The model under review builds one solid part; all positions refer to its coordinate system, in mm. A direction names the side the tool comes from. Round coordinates to 2 decimals unless told otherwise and drop trailing zeros. Order: outer loops, then holes, each group sorted by start corner. A loop starts at its lowest first (then second) coordinate and runs counter-clockwise, first axis right, second up. Notation, with made-up numbers: M 35.5,65 L 68.5,65 A10 ccw 68.5,81 Z; hole C 46.25,52 d9. An arc over 180 degrees is marked long. Answer as a JSON object with one key per item and string values. Group by question number.
1. Clearance check with flat-ended pins moving along their axes: P1, Ø2.5, axis at x = 14, z = 5.5, coming from the +Y side; P2, Ø10, axis at x = -13.5, z = 5.5, coming from the +Y side; P3, Ø8.5, axis at x = 12, z = -3, coming from the +Y side. State where each tip first meets the part, or that it passes through.
2. To check wall thickness, follow probe 1 along X at (y, z) = (1.75, 6.75); probe 2 along Z at (x, y) = (21, 1.5); probe 3 along Y at (x, z) = (-6.5, 7.5). State the ranges of each line that lie inside material, in increasing order. Write a range as [from, to].
3. Add section C-C on y = 3. Give the number of separate pieces and of enclosed holes in the cut face, and give its area (3 significant figures).
4. Add section B-B on z = -5. State the section outline as (x, y) points, and give its area (3 significant figures).
5. Add section A-A on x = -6. State the section outline as (y, z) points, and give its area (3 significant figures).
6. Machinability: for faces 1 (the face through (11, 0.5, -4)), 2 (the face through (22.21, 0.99, 8.23)), 3 (the face through (-0.218, 3.288, -1.663)), which of the approach directions +Z, -Z, +X, -X, +Y, -Y give a long, thin tool a straight path to every point of the face, cutting with its end or side? Answer none if there is none.
7. Mouldability with a two-part tool opening along Z and no side actions: class faces 4 (the face through (-22.21, 0.99, -8.23)), 5 (the face through (0, 0, 0)), 6 (the face through (-22.4, 3, 8.3)), 7 (the face through (-1.375, 3.288, 1.35)) as released by +Z, released by -Z, zero draft, split by the parting line, or undercut.
```python
from build123d import *

# Parameters (mm, degrees)
BOSS_EXTRUDE1_DEPTH = 4
BOSS_EXTRUDE1_DRAFT = -1
SHELL1_T            = -0.5
SKETCH2_R           = 2
BOSS_EXTRUDE2_DEPTH = 5.5
BOSS_EXTRUDE2_TAPER = 1.5
CIRPATTERN1_COUNT   = 4
SKETCH4_R           = 1.605977431
CUT_EXTRUDE1_DEPTH  = 5.5
CUT_EXTRUDE1_DRAFT  = 1.5
RIB3_START          = -22.069744096
RIB3_DEPTH          = 20.231981802
RIB3_START_2        = 1.837762294
RIB3_2_DEPTH        = 20.231981802
RIB3_START_3        = -8.069744096
RIB3_3_DEPTH        = 6.231981802
RIB3_4_DEPTH        = 6.231981802


with BuildPart() as part:
    # Sketch1 → Boss-Extrude1 (with draft: the straight prism first)
    with BuildSketch(Plane(origin=(0, 0, 0), x_dir=(1, 0, 0), z_dir=(0, 1, 0))):
        with BuildLine():
            Line((-21.5, -8.5), (21.5, -8.5))
            ThreePointArc((21.5, -8.5), (22.207106781, -8.207106781), (22.5, -7.5))
            Line((22.5, -7.5), (22.5, 7.5))
            ThreePointArc((22.5, 7.5), (22.207106781, 8.207106781), (21.5, 8.5))
            Line((21.5, 8.5), (-21.5, 8.5))
            ThreePointArc((-21.5, 8.5), (-22.207106781, 8.207106781), (-22.5, 7.5))
            Line((-22.5, 7.5), (-22.5, -7.5))
            ThreePointArc((-22.5, -7.5), (-22.207106781, -8.207106781), (-21.5, -8.5))
        make_face()
    extrude(amount=BOSS_EXTRUDE1_DEPTH)
    # Boss-Extrude1: the draft: its side faces are tilted about the plane it starts from
    boss_extrude1_sides = [part.faces().sort_by_distance(p)[0] for p in [
        (0, 2, 8.5),
        (22.207106781, 2, 8.207106781),
        (22.5, 2, 0),
        (22.207106781, 2, -8.207106781),
        (0, 2, -8.5),
        (-22.207106781, 2, -8.207106781),
        (-22.5, 2, 0),
        (-22.207106781, 2, 8.207106781),
    ]]
    draft(boss_extrude1_sides, Plane(origin=(0, 0, 0), x_dir=(1, 0, 0), z_dir=(0, 1, 0)), BOSS_EXTRUDE1_DRAFT)

    # Shell1
    shell1_openings = [part.faces().sort_by_distance(p)[0] for p in [
        (0, 4, 0),
    ]]
    offset(amount=SHELL1_T, openings=shell1_openings, kind=Kind.INTERSECTION)

    # Sketch2 → Boss-Extrude2 (add)
    with BuildSketch(Plane(origin=(0, 0.5, 0), x_dir=(1, 0, 0), z_dir=(0, 1, 0))):
        Circle(SKETCH2_R)
    extrude(amount=BOSS_EXTRUDE2_DEPTH, taper=BOSS_EXTRUDE2_TAPER)

    # Rib2: read off the stored shape, not the designer's step
    # Rib2: loft between two sections, ruled curve by curve
    rib2_from = [
        Edge.make_line((1.837762394, 6, 0.25938699), (2.378960183, 6, 0.25)),
        Edge.make_line((1.837762394, 6, -0.25938699), (2.378960183, 6, -0.25)),
        Edge.make_line((2.378960183, 6, -0.25), (2.378960183, 6, 0.25)),
        Edge.make_line((1.837762394, 6, -0.25938699), (1.837762394, 6, 0.25938699)),
    ]
    rib2_to = [
        Edge.make_line((1.982009028, 0.5, 0.267656891), (3, 0.5, 0.25)),
        Edge.make_line((1.982009028, 0.5, -0.267656891), (3, 0.5, -0.25)),
        Edge.make_line((3, 0.5, -0.25), (3, 0.5, 0.25)),
        Edge.make_line((1.982009028, 0.5, -0.267656891), (1.982009028, 0.5, 0.267656891)),
    ]
    rib2 = Solid(Shell([*[Face.make_surface_from_curves(rib2_from[k], rib2_to[k]) for k in range(4)], Face(Wire(rib2_from)), Face(Wire(rib2_to))]))
    add(rib2)

    # CirPattern1: Rib2 ×4 about axis
    cirpattern1_axis = Axis((0, 0, 0), (0, 1, 0))
    for i in range(1, CIRPATTERN1_COUNT):
        add(rib2.rotate(cirpattern1_axis, i * 360 / CIRPATTERN1_COUNT))


with BuildPart() as cut_extrude1_tool:
    # Sketch4 → Cut-Extrude1 (with draft: the straight prism first)
    with BuildSketch(Plane(origin=(0, 6, 0), x_dir=(1, 0, 0), z_dir=(0, 1, 0))):
        Circle(SKETCH4_R)
    extrude(amount=-CUT_EXTRUDE1_DEPTH)
    # Cut-Extrude1: the draft: its side faces are tilted about the plane it starts from
    cut_extrude1_sides = [cut_extrude1_tool.faces().sort_by_distance(p)[0] for p in [
        (-1.605977431, 3.25, 0),
    ]]
    draft(cut_extrude1_sides, Plane(origin=(0, 6, 0), x_dir=(1, 0, 0), z_dir=(0, 1, 0)), CUT_EXTRUDE1_DRAFT)


with BuildPart() as part_1:
    add(part.part)

    # Cut-Extrude1: cut by cut_extrude1_tool
    add(cut_extrude1_tool.part, mode=Mode.SUBTRACT)

    # Rib3: read off the stored shape, not the designer's step
    # Rib3 outline → Rib3 (add)
    with BuildSketch(Plane.YZ.offset(RIB3_START)):
        Polygon((0.5, -0.276182597), (2, -0.25), (2, 0.25), (0.5, 0.276182597), align=None)
    extrude(amount=RIB3_DEPTH)

    # Rib3 2 outline → Rib3 2 (add)
    with BuildSketch(Plane.YZ.offset(RIB3_START_2)):
        Polygon((0.5, -0.276182597), (2, -0.25), (2, 0.25), (0.5, 0.276182597), align=None)
    extrude(amount=RIB3_2_DEPTH)

    # Rib3 3 outline → Rib3 3 (add)
    with BuildSketch(Plane.XY.offset(RIB3_START_3)):
        Polygon((0.276182597, 0.5), (0.25, 2), (-0.25, 2), (-0.276182597, 0.5), align=None)
    extrude(amount=RIB3_3_DEPTH)

    # Rib3 4 outline → Rib3 4 (add)
    with BuildSketch(Plane.XY.offset(RIB3_START_2)):
        Polygon((0.276182597, 0.5), (0.25, 2), (-0.25, 2), (-0.276182597, 0.5), align=None)
    extrude(amount=RIB3_4_DEPTH)

    # Sweep1: sweep along a path in Sketch8
    with BuildLine(Plane(origin=(0, 2, 0), x_dir=(-1, 0, 0), z_dir=(0, -1, 0))) as sweep1_path:
        Line((22.56982026, 7.5), (22.56982026, -7.5))
        ThreePointArc((22.56982026, -7.5), (22.25647716, -8.25647716), (21.5, -8.56982026))
        Line((21.5, -8.56982026), (-21.5, -8.56982026))
        ThreePointArc((-21.5, -8.56982026), (-22.25647716, -8.25647716), (-22.56982026, -7.5))
        Line((-22.56982026, -7.5), (-22.56982026, 7.5))
        ThreePointArc((-22.56982026, 7.5), (-22.25647716, 8.25647716), (-21.5, 8.56982026))
        Line((-21.5, 8.56982026), (21.5, 8.56982026))
        ThreePointArc((21.5, 8.56982026), (22.25647716, 8.25647716), (22.56982026, 7.5))
    # Sketch5 → Sweep1 (sweep)
    with BuildSketch(Plane(origin=(0, 0, 0), x_dir=(0, 0, -1), z_dir=(1, 0, 0))):
        Polygon((-8.83491013, 2), (-8.56982026, 4), (-8.53491013, 2), align=None)
    sweep(path=sweep1_path.line)


solid = part_1.part
```
Recorded:
{
 "1": {"P1": "stops at y = 0.5", "P2": "stops at y = 4", "P3": "stops at y = 2"},
 "2": {"probe 1": "x = [-22.53, -22.03], [-0.25, 0.25], [22.03, 22.53]", "probe 2": "z = [-8.53, -8.03], [-0.26, 0.26], [8.03, 8.53]", "probe 3": "y = [0, 0.5]"},
 "3": {"separate pieces": "2", "enclosed holes": "2", "area": "83.5 mm²"},
 "4": {"outline": "M -22.83,2 L -22.53,2 L -22.5,0 L 22.5,0 L 22.53,2 L 22.83,2 L 22.57,4 L 22.07,4 L 22.01,0.5 L 0.28,0.5 L 0.25,2 L -0.25,2 L -0.28,0.5 L -22.01,0.5 L -22.07,4 L -22.57,4 Z", "area": "27.4 mm²"},
 "5": {"outline": "M 0,-8.5 L 2,-8.53 L 2,-8.83 L 4,-8.57 L 4,-8.07 L 0.5,-8.01 L 0.5,-0.28 L 2,-0.25 L 2,0.25 L 0.5,0.28 L 0.5,8.01 L 4,8.07 L 4,8.57 L 2,8.83 L 2,8.53 L 0,8.5 Z", "area": "13.4 mm²"},
 "6": {"face 1": "+Y", "face 2": "+Z, +X, -Y", "face 3": "none"},
 "7": {"face 4": "released by -Z", "face 5": "zero draft", "face 6": "released by +Z", "face 7": "undercut"}
}
